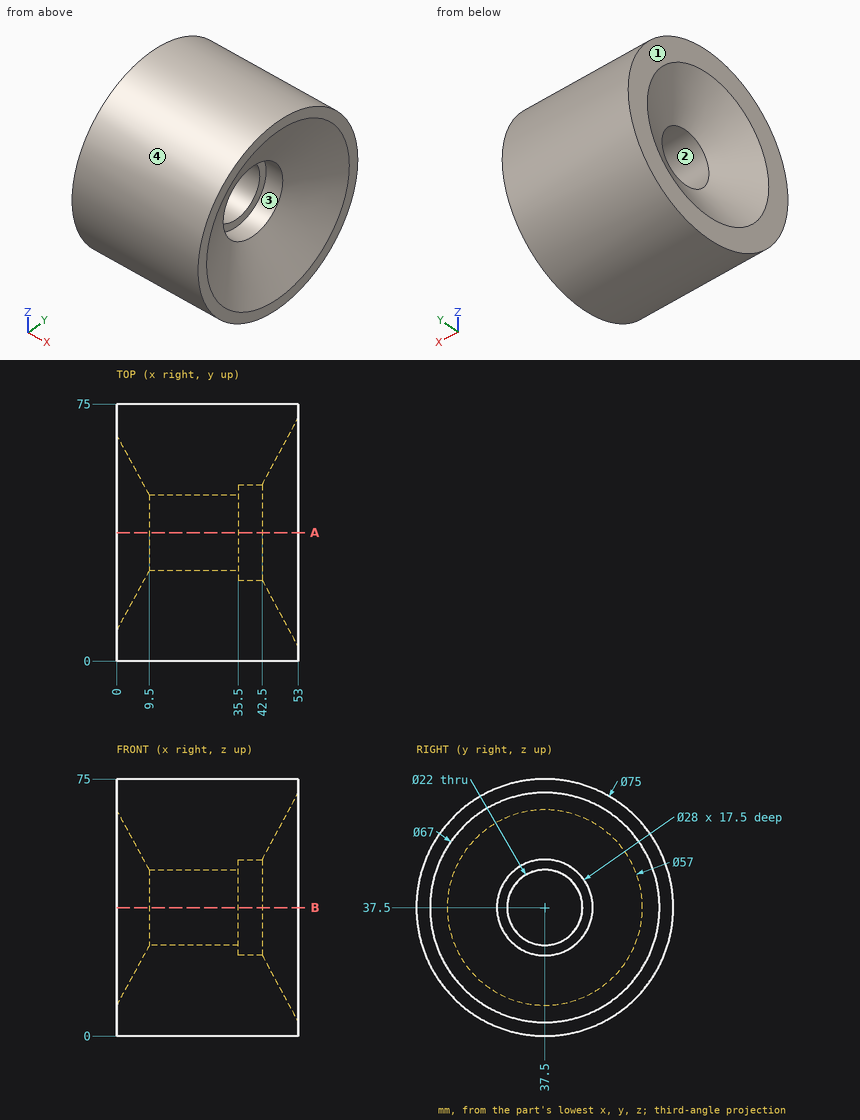
Source: three-view drawing plus pictorial views. Frame: mm from the lowest corner of the part. Give positions to 0.01 mm unless a question says otherwise; leave off trailing zeros. Order: outer loops, then holes, each group sorted by start corner. A loop starts at its lowest first (then second) coordinate and runs counter-clockwise, first axis right, second up. Notation, with made-up numbers: (23.5, 74.25) -> (81.5, 74.25) arc R14 cw to (81.5, 93.25) -> close; hole circle Ø11 at (-11.75, -35). An arc over 180 degrees is marked (long way). Use a Markdown table: item, result.
Q1. Section A-A (y = 37.5). Return the cut outline in (x, z).
A:
| item | result |
|---|---|
| outline | (0, 0) -> (53, 0) -> (53, 4) -> (42.5, 23.5) -> (35.5, 23.5) -> (35.5, 26.5) -> (9.5, 26.5) -> (0, 9) -> close; (0, 66) -> (9.5, 48.5) -> (35.5, 48.5) -> (35.5, 51.5) -> (42.5, 51.5) -> (53, 71) -> (53, 75) -> (0, 75) -> close |
Q2. Material intervals for line 1 (Y direction, x = 20, z = 37); line 2 (Z direction, x = 38.5, y = 37.5); line 3 (X direction, y = 22, z = 64), sorted ascending. Write a range as [from, to].
A:
| item | result |
|---|---|
| line 1 | [0, 26.51], [48.49, 75] |
| line 2 | [0, 23.5], [51.5, 75] |
| line 3 | [0, 51.49] |
Q3. First-contact query: P1, Ø10, axis at x = 25.5, z = 53, coming from the -Y side; P2, Ø8, axis at x = 36, z = 55, coming from the +Y side; P3, Ø1.5, axis at x = 12, y = 59, coming from the -Z side; P4, Ø1.5, axis at y = 25, z = 64, coming from the -X side. Flat tips, straight axial feed; report the tip coordinate or a pass-through.
A:
| item | result |
|---|---|
| P1 | y = 1.5 |
| P2 | y = 72.49 |
| P3 | z = 6.26 |
| P4 | x = 0 |
Q4. Pull-direction query (Y, two-part tool) for the marked faces 1, 2, 3 and 4; classes: +Y half, -Y half, draft (parallel to the pull), parting line (faces both ways), or undercut.
A:
| item | result |
|---|---|
| face 1 | draft |
| face 2 | undercut |
| face 3 | undercut |
| face 4 | parting line |
